Here's how the part is built. I have some questions about the finished solid (model axes, mm). A direction names the side the tool comes from. Coordinates: 2 decimals unless noted, no trailing zeros. Write each loop counter-clockwise with the first axis right and the second up, starting at its lowest first coordinate (ties: lowest second). Pieces come first, ordered by that corner, then holes. Notation, with made-up numbers: M -12,-28 L 31,-28 A19 ccw 31,-19 Z; hole C 68,-27.75 d11. An arc over 180 degrees is marked long. Use a Markdown table: item, result.
```python
from build123d import *

# Parameters (mm, degrees)
BOSS_EXTRUDE1_DEPTH  = 60
SKETCH3_R            = 2
CUT_EXTRUDE2_DEPTH   = 35
SKETCH2_W            = 117.6
SKETCH2_H            = 50
CUT_EXTRUDE4_DEPTH   = 55
BOSS_EXTRUDE2_DEPTH  = 50
SKETCH8_R            = 12.7
CUT_EXTRUDE5_DEPTH   = 35
SKETCH13_R           = 2
CUT_EXTRUDE6_DEPTH   = 145.190091546
SKETCH14_R           = 1.5
CUT_EXTRUDE7_DEPTH   = 10
SKETCH16_R           = 12.5
CUT_EXTRUDE8_DEPTH   = 10
SKETCH17_R           = 1.5
CUT_EXTRUDE9_DEPTH   = 20
SKETCH18_R           = 1.5
CUT_EXTRUDE10_DEPTH  = 20
LPATTERN1_COUNT      = 4
LPATTERN1_PITCH      = 35
LPATTERN1_COUNT_DIR2 = 2
LPATTERN1_PITCH_DIR2 = 55
FILLET1_R            = 10


with BuildPart() as part:
    # Sketch1 → Boss-Extrude1 (new body)
    with BuildSketch(Plane.XY):
        with BuildLine():
            Line((-58.8, -30.15), (58.8, -30.15))
            ThreePointArc((58.8, -30.15), (62.335533906, -28.685533906), (63.8, -25.15))
            Line((63.8, -25.15), (63.8, 24.85))
            ThreePointArc((63.8, 24.85), (62.335533906, 28.385533906), (58.8, 29.85))
            Line((58.8, 29.85), (-58.8, 29.85))
            ThreePointArc((-58.8, 29.85), (-62.335533906, 28.385533906), (-63.8, 24.85))
            Line((-63.8, 24.85), (-63.8, -25.15))
            ThreePointArc((-63.8, -25.15), (-62.335533906, -28.685533906), (-58.8, -30.15))
        make_face()
        with BuildLine():
            Line((53.8, 5.15), (12.8, 5.15))
            ThreePointArc((12.8, 5.15), (11.385786438, 4.564213562), (10.8, 3.15))
            Line((10.8, 3.15), (10.8, -3.15))
            ThreePointArc((10.8, -3.15), (11.385786438, -4.564213562), (12.8, -5.15))
            Line((12.8, -5.15), (53.8, -5.15))
            ThreePointArc((53.8, -5.15), (55.214213562, -4.564213562), (55.8, -3.15))
            Line((55.8, -3.15), (55.8, 3.15))
            ThreePointArc((55.8, 3.15), (55.214213562, 4.564213562), (53.8, 5.15))
        make_face(mode=Mode.SUBTRACT)
    extrude(amount=BOSS_EXTRUDE1_DEPTH)

    # Sketch3 → Cut-Extrude2 (cut)
    with BuildSketch(Plane.XY.offset(60)):
        with Locations((14.3, 16.85)):
            Circle(SKETCH3_R)
        with Locations((34.3, 16.85)):
            Circle(SKETCH3_R)
        with Locations((54.3, 16.85)):
            Circle(SKETCH3_R)
        with Locations((34.3, -17.15)):
            Circle(SKETCH3_R)
        with Locations((54.3, -17.15)):
            Circle(SKETCH3_R)
        with Locations((14.3, -17.15)):
            Circle(SKETCH3_R)
    extrude(amount=-CUT_EXTRUDE2_DEPTH, mode=Mode.SUBTRACT)

    # Sketch2 → Cut-Extrude4 (cut)
    with BuildSketch(Plane(origin=(0, 0, 0), x_dir=(-1, 0, 0), z_dir=(0, 0, -1))):
        with Locations((0, -0.15)):
            Rectangle(SKETCH2_W, SKETCH2_H)
    extrude(amount=-CUT_EXTRUDE4_DEPTH, mode=Mode.SUBTRACT)

    # Sketch12 → Boss-Extrude2 (add)
    with BuildSketch(Plane(origin=(0, 0, 55), x_dir=(-1, 0, 0), z_dir=(0, 0, -1))):
        Polygon((53.8, 24.85), (38.80387838, 24.85), (38.80387838, -25.15), (58.8, -25.15), (58.8, 19.85), (58.8, 24.85), align=None)
    extrude(amount=BOSS_EXTRUDE2_DEPTH)

    # Sketch8 → Cut-Extrude5 (cut)
    with BuildSketch(Plane.ZY.offset(63.8)):
        with Locations(Location((30, -0.15, 0), (0, 0, 270))):
            Circle(SKETCH8_R)
    extrude(amount=-CUT_EXTRUDE5_DEPTH, mode=Mode.SUBTRACT)

    # Sketch13 → Cut-Extrude6 (cut, through all)
    with BuildSketch(Plane.ZY.offset(63.8)):
        with Locations((10, -19.15)):
            Circle(SKETCH13_R)
        with Locations((50, 19.85)):
            Circle(SKETCH13_R)
    extrude(amount=-CUT_EXTRUDE6_DEPTH, mode=Mode.SUBTRACT)

    # Sketch14 → Cut-Extrude7 (cut)
    with BuildSketch(Plane(origin=(0, 0, 5), x_dir=(-1, 0, 0), z_dir=(0, 0, -1))):
        with Locations((52.64387838, -0.15)):
            Circle(SKETCH14_R)
        with Locations((42.04387838, 15.05)):
            Circle(SKETCH14_R)
        with Locations((42.04387838, -15.35)):
            Circle(SKETCH14_R)
    extrude(amount=-CUT_EXTRUDE7_DEPTH, mode=Mode.SUBTRACT)

    # Sketch16 → Cut-Extrude8 (cut)
    with BuildSketch(Plane(origin=(56.19612162, 0, 0), x_dir=(0, 0, -1), z_dir=(1, 0, 0))):
        with Locations((-30, -0.15)):
            Circle(SKETCH16_R)
    extrude(amount=CUT_EXTRUDE8_DEPTH, mode=Mode.SUBTRACT)

    # Sketch17 → Cut-Extrude9 (cut)
    with BuildSketch(Plane(origin=(0, 0, 0), x_dir=(-1, 0, 0), z_dir=(0, 0, -1))):
        with Locations((-53.8, 27.35)):
            Circle(SKETCH17_R)
    cut_extrude9 = extrude(amount=-CUT_EXTRUDE9_DEPTH, mode=Mode.SUBTRACT)

    # Sketch18 → Cut-Extrude10 (cut)
    with BuildSketch(Plane(origin=(0, 0, 0), x_dir=(-1, 0, 0), z_dir=(0, 0, -1))):
        with Locations((-61.3, 9.85)):
            Circle(SKETCH18_R)
        with Locations((-61.3, -10.15)):
            Circle(SKETCH18_R)
    cut_extrude10 = extrude(amount=-CUT_EXTRUDE10_DEPTH, mode=Mode.SUBTRACT)

    # LPattern1: Cut-Extrude9 4 × 2
    with Locations(*[(-i * LPATTERN1_PITCH, -j * LPATTERN1_PITCH_DIR2, 0) for i in range(LPATTERN1_COUNT) for j in range(LPATTERN1_COUNT_DIR2) if (i, j) != (0, 0)]):
        add(cut_extrude9, mode=Mode.SUBTRACT)

    # Mirror1: Cut-Extrude10 across plane
    add(cut_extrude10.mirror(Plane(origin=(0, 0, 0), x_dir=(0, 0, 1), z_dir=(1, 0, 0))), mode=Mode.SUBTRACT)

    # Fillet1
    # the kernel refuses this fillet: 10 mm, written as the material it adds along each edge
    with BuildSketch(Plane(origin=(-38.80387838, 24.85, 55), x_dir=(1, 0, 0), z_dir=(0, 0, -1))) as fillet1_piece_1_section:
        with BuildLine():
            CenterArc((FILLET1_R, FILLET1_R), FILLET1_R, 180, 90)
            Line((0, FILLET1_R), (0, 0))
            Line((0, 0), (FILLET1_R, 0))
        make_face()
    fillet1_piece_1 = extrude(amount=50, mode=Mode.PRIVATE)
    fillet1_piece_1 = fillet1_piece_1 - Plane(origin=(-36.514873335, 19.85, 50), x_dir=(0, 0, 1), z_dir=(-1, 0, 0)) * Cylinder(2, 140, mode=Mode.PRIVATE)
    add(fillet1_piece_1)
    with BuildSketch(Plane(origin=(-38.80387838, -25.15, 55), x_dir=(1, 0, 0), z_dir=(0, 0, -1))) as fillet1_piece_2_section:
        with BuildLine():
            CenterArc((FILLET1_R, -FILLET1_R), FILLET1_R, 90, 90)
            Line((0, -FILLET1_R), (0, 0))
            Line((0, 0), (FILLET1_R, 0))
        make_face()
    fillet1_piece_2 = extrude(amount=50, mode=Mode.PRIVATE)
    fillet1_piece_2 = fillet1_piece_2 - Plane(origin=(-36.519941054, -19.15, 10), x_dir=(0, 0, 1), z_dir=(-1, 0, 0)) * Cylinder(2, 140, mode=Mode.PRIVATE)
    add(fillet1_piece_2)
    with BuildSketch(Plane(origin=(58.8, 24.85, 0), x_dir=(-1, 0, 0), z_dir=(0, 0, 1))) as fillet1_piece_3_section:
        with BuildLine():
            CenterArc((FILLET1_R, FILLET1_R), FILLET1_R, 180, 90)
            Line((0, FILLET1_R), (0, 0))
            Line((0, 0), (FILLET1_R, 0))
        make_face()
    fillet1_piece_3 = extrude(amount=55, mode=Mode.PRIVATE)
    fillet1_piece_3 = fillet1_piece_3 - Plane(origin=(56.513305824, 19.85, 50), x_dir=(0, 0, 1), z_dir=(-1, 0, 0)) * Cylinder(2, 150, mode=Mode.PRIVATE)
    add(fillet1_piece_3)
    with BuildSketch(Plane(origin=(58.8, -25.15, 0), x_dir=(0, 1, 0), z_dir=(0, 0, 1))) as fillet1_piece_4_section:
        with BuildLine():
            CenterArc((FILLET1_R, FILLET1_R), FILLET1_R, 180, 90)
            Line((0, FILLET1_R), (0, 0))
            Line((0, 0), (FILLET1_R, 0))
        make_face()
    fillet1_piece_4 = extrude(amount=55, mode=Mode.PRIVATE)
    fillet1_piece_4 = fillet1_piece_4 - Plane(origin=(56.517896766, -19.15, 10), x_dir=(0, 0, 1), z_dir=(-1, 0, 0)) * Cylinder(2, 150, mode=Mode.PRIVATE)
    add(fillet1_piece_4)


solid = part.part
```
1. Suppose I cut it at A-A on y = -0.15. Write out the boundary of the cut face in (x, z), and give its area (3 significant figures).
Answers follow:
| item | result |
|---|---|
| outline | M -63.8,0 L -58.8,0 L -58.8,5 L -54.14,5 L -54.14,15 L -51.14,15 L -51.14,5 L -38.8,5 L -38.8,17.3 L -63.8,17.3 Z; M -63.8,42.7 L -38.8,42.7 L -38.8,55 L 10.8,55 L 10.8,60 L -63.8,60 Z; M 55.8,55 L 58.8,55 L 58.8,42.5 L 63.8,42.5 L 63.8,60 L 55.8,60 Z; M 58.8,0 L 63.8,0 L 63.8,17.5 L 58.8,17.5 Z |
| area | 1,170 mm2 |
2. Suppose I cut it at D-D on z = 13.5. State how many separate pieces and enclosed holes the cut face has, and give its area (3 significant figures).
Answers follow:
| item | result |
|---|---|
| separate pieces | 1 |
| enclosed holes | 16 |
| area | 2,730 mm2 |
3. We'd pull the mould along X, two halves only. Please class faces 4 (the face through (0, 27, 0)), 5 (the face through (-62.37, -28.65, 29.58)), 6 (the face through (8, 24.85, 27)): +X half, -X half, draft (parallel to the pull), parting line (faces both ways), or undercut.
Answers follow:
| item | result |
|---|---|
| face 4 | draft |
| face 5 | -X half |
| face 6 | undercut |
4. Which directions (+Z, -Z, +X, -X, +Y, -Y) give clear straight access to the entire face, cutting with the end or side of a thin tool? Please do faces 1 (the face through (-15.875, 25.886, 9.86)), 2 (the face through (63.8, -12, 23)), 3 (the face through (10.8, 0, 57)).
Answers follow:
| item | result |
|---|---|
| face 1 | -Z |
| face 2 | +Z, -Z, +X, +Y, -Y |
| face 3 | +Z, -Z |
5. Will these pins go through, and if not, where does the flat tip stop? pin 1 Ø22.5 at (y, z) = (-0.15, 30) entering from -X (3 decimals); pin 2 Ø4 at (x, y) = (-15.5, -21) entering from -Z; pin 3 Ø0.9 at (x, y) = (-51.5, 26.5) entering from -Z; pin 4 Ø2.5 at (x, y) = (-42, -15.5) entering from -Z.
Answers follow:
| item | result |
|---|---|
| pin 1 | passes through |
| pin 2 | stops at z = 55 |
| pin 3 | stops at z = 20 |
| pin 4 | stops at z = 15 |
6. Suppose I cut it at C-C on z = 46.5. Write out the boundary of the cut face in (x, y), and give its area (3 significant figures).
Answers follow:
| item | result |
|---|---|
| outline | M -63.8,-25.15 A5 ccw -58.8,-30.15 L 58.8,-30.15 A5 ccw 63.8,-25.15 L 63.8,24.85 A5 ccw 58.8,29.85 L -58.8,29.85 A5 ccw -63.8,24.85 Z; hole M -38.8,-15.15 A10 ccw -28.8,-25.15 L 48.8,-25.15 A10 ccw 58.8,-15.15 L 58.8,14.85 A10 ccw 48.8,24.85 L -28.8,24.85 A10 ccw -38.8,14.85 Z |
| area | 2,840 mm2 |
7. I need wall thicknesses on probe 1 along Y at (x, z) = (14.3, 56.8); probe 2 along Y at (x, z) = (54, 57); probe 3 along Z at (x, y) = (61.35, -0.15). Which ranges of each line are inside material? Lowest first, please.
Answers follow:
| item | result |
|---|---|
| probe 1 | y = -30.15 to -19.15, -15.15 to -5.15, 5.15 to 14.85, 18.85 to 29.85 |
| probe 2 | y = -30.15 to -19.13, -15.17 to -5.14, 5.14 to 14.87, 18.83 to 29.85 |
| probe 3 | z = 0 to 17.5, 42.5 to 60 |
8. Suppose I cut it at B-B on x = 14.3. Write out the boundary of the cut face in (y, z), and give its area (4 significant figures).
Answers follow:
| item | result |
|---|---|
| outline | M -30.15,0 L -25.15,0 L -25.15,55 L -19.15,55 L -19.15,60 L -30.15,60 Z; M -15.15,55 L -5.15,55 L -5.15,60 L -15.15,60 Z; M 5.15,55 L 14.85,55 L 14.85,60 L 5.15,60 Z; M 18.85,55 L 24.85,55 L 24.85,0 L 29.85,0 L 29.85,60 L 18.85,60 Z |
| area | 758.5 mm2 |
